from build123d import *

# Parameters (mm, degrees)
EXTRUDE_START       = -22
EXTRUDE_SKETCH_1_R  = 5
EXTRUDE_1_DEPTH     = 52
EXTRUDE_START_2     = 26
EXTRUDE_SKETCH_2_R  = 9
EXTRUDE_2_DEPTH     = 6
PIPE_SKETCH_1_R     = 4.5
PIPE_1_DEPTH        = 48
PIPE_ROTATE_1_ANGLE = 90
EXTRUDE_START_3     = 30
EXTRUDE_SKETCH_3_R  = 4.5
EXTRUDE_3_DEPTH     = 8


with BuildPart() as part:
    # Extrude sketch 1 → Extrude 1 (new body)
    with BuildSketch(Plane.XY.offset(EXTRUDE_START)):
        Circle(EXTRUDE_SKETCH_1_R)
    extrude(amount=EXTRUDE_1_DEPTH)


with BuildPart() as body_2:
    # Extrude sketch 2 → Extrude 2 (new body)
    with BuildSketch(Plane.XY.offset(EXTRUDE_START_2)):
        Circle(EXTRUDE_SKETCH_2_R)
    extrude(amount=EXTRUDE_2_DEPTH)


with BuildPart() as body_3:
    # Pipe sketch 1 → Pipe 1 (new body)
    with BuildSketch(Plane.XY):
        Circle(PIPE_SKETCH_1_R)
    extrude(amount=PIPE_1_DEPTH)


with BuildPart() as body_3_1:
    # Pipe rotate 1: moved
    add(body_3.part.rotate(Axis((0, 0, 0), (0, 1, 0)), PIPE_ROTATE_1_ANGLE))


with BuildPart() as body_3_2:
    # Pipe place 1: moved
    add(body_3_1.part.moved(Location((-24, 0, 38))))


with BuildPart() as body_4:
    # Extrude sketch 3 → Extrude 3 (new body)
    with BuildSketch(Plane.XY.offset(EXTRUDE_START_3)):
        Circle(EXTRUDE_SKETCH_3_R)
    extrude(amount=EXTRUDE_3_DEPTH)


with BuildPart() as body_3_3:
    add(body_3_2.part)

    # Combine (weld / assembly of features): union body 2, body 4, part
    add(body_2.part)
    add(body_4.part)
    add(part.part)


solid = body_3_3.part
Model file for the job. Use its own axes, mm. A direction names the side the tool comes from. Round coordinates to 2 decimals unless told otherwise and drop trailing zeros. Loops run counter-clockwise (first coordinate to the right, second up) from the corner with the lowest first, then second, coordinate; pieces in that order, holes last. Notation, with made-up numbers: (8.5, 22) -> (42.5, 22) arc R16 cw to (42.5, 27) -> close; hole circle Ø6 at (51, 51). An arc over 180 degrees is marked (long way). Answer as CSV lines item,"result". Start each with the question number.
1) Pin check, flat tips, straight feed: P1, Ø5, axis at x = 6, z = 32, coming from the -Y side; P2, Ø4, axis at y = 4, z = 5, coming from the -X side; P3, Ø8, axis at y = 2.5, z = -13, coming from the -X side. Stop position of each tip, or through.
2) Mould opens along Z. For faces 4 (the face through (0, 0, -22)), 5 (the face through (-1.08, -4.88, 1.66)), 6 (the face through (2.08, -3.99, 33.62)) say: +Z half, -Z half, draft (parallel to the pull), parting line (faces both ways), or undercut.
3) Slice it at A-A (x = 0). List the corners of the cut face in (y, z), plus the area to 3 significant figures.
4) Slice it at D-D (z = 37). List the corners of the cut face in (x, y).
5) Probe line 1 along Z through (x, y) = (13.5, 0.25); line 2 along Z through (x, y) = (0, 7); line 3 along X through (y, z) = (0.25, -19). List the from-to ranges inside material, lowest first.
6) Slice it at B-B (y = 0). List the corners of the cut face in (x, z), plus the area to 3 significant figures.
7) Slice it at C-C (z = 27). List the corners of the cut face in (x, y), plus the area to 3 significant figures.
8) Tool access for faces 1 (the face through (-1.172, 8.923, 28.958)), 2 (the face through (24, 0, 38)), 3 (the face through (-0.336, 0.198, 42.496)): list every direction of +Z, -Z, +X, -X, +Y, -Y with a clear straight run to the whole face (end or side of a thin tool).
Filled in:
1,P1,"stops at y = -8.29"
1,P2,"stops at x = -4.58"
1,P3,"stops at x = -5"
2,face 4,"-Z half"
2,face 5,"draft"
2,face 6,"undercut"
3,outline,"(-9, 26) -> (-5, 26) -> (-5, -22) -> (5, -22) -> (5, 26) -> (9, 26) -> (9, 32) -> (4.5, 32) -> (4.5, 38) arc R4.5 ccw to (-4.5, 38) -> (-4.5, 32) -> (-9, 32) -> close"
3,area,"674 mm2"
4,outline,"(-24, -4.39) -> (-1, -4.39) arc R4.5 ccw to (1, -4.39) -> (24, -4.39) -> (24, 4.39) -> (1, 4.39) arc R4.5 ccw to (-1, 4.39) -> (-24, 4.39) -> close"
5,line 1,"z = 33.51 to 42.49"
5,line 2,"z = 26 to 32"
5,line 3,"x = -4.99 to 4.99"
6,outline,"(-24, 33.5) -> (-4.5, 33.5) -> (-4.5, 32) -> (-9, 32) -> (-9, 26) -> (-5, 26) -> (-5, -22) -> (5, -22) -> (5, 26) -> (9, 26) -> (9, 32) -> (4.5, 32) -> (4.5, 33.5) -> (24, 33.5) -> (24, 42.5) -> (-24, 42.5) -> close"
6,area,"1,030 mm2"
7,outline,"circle Ø18 at (0, 0)"
7,area,"254 mm2"
8,face 1,"-Z"
8,face 2,"+Z, -Z, +X, +Y, -Y"
8,face 3,"none"
